Geometry check sheet. Reference: the model listing, model coordinates, mm. Coordinates: 2 decimals unless noted, no trailing zeros. Write each loop counter-clockwise with the first axis right and the second up, starting at its lowest first coordinate (ties: lowest second). Pieces come first, ordered by that corner, then holes. Notation, with made-up numbers: M 71,37 L 117,37 A15 ccw 117,61 Z; hole C -30,52 d7. An arc over 180 degrees is marked long. Put each result on its own line as item: value. Start each with the question number.
1) Cross-section at A-A on z = 0. Record the cut outline in (x, y) (3 decimals), plus the area to 3 significant figures.
2) Gauge pin test, flat ends, axial feed: pin 1 (8 mm diameter, centred on x = 1, y = -21, fed in from -Z); pin 2 (8 mm diameter, centred on x = -5.5, y = -5.5, fed in from -Z); pin 3 (12 mm diameter, centred on y = 16, z = 39, fed in from -X); pin 4 (3 mm diameter, centred on x = -15.5, z = -24.5, fed in from +Y). Record the tip position at first contact, or that the pin passes through.
3) Scan lines: line 1 along Z through (x, y) = (8, 0) (3 decimals); line 2 along Z through (x, y) = (15, -38.5); line 3 along Y through (x, z) = (12.5, 23.5). Record each from-to range of solid material in increasing order.
4) Mould release check, pull along Z, two halves, no side actions. Record for faces 1 (the flat face through (27, 22, -41)), 2 (the cylindrical face through (-0.36, -35.81, -27.46)), 3 (the conical face through (-26.854, -10.915, -49.155)): released by +Z, released by -Z, zero draft, split by the parting line, or undercut.
5) Cross-section at C-C on x = -11. Record the cut outline in (y, z) (3 decimals), plus the area to 3 significant figures.
from build123d import *

# Parameters (mm, degrees)
F0_R     = 52
F0_R_2   = 45.125
F1_DEPTH = 27
F2_SIZE  = 1
F3_SIZE2 = 1.7320508076
F3_SIZE  = 3


with BuildPart() as f1:
    # F0 (on Right) → F1 (new body, symmetric)
    with BuildSketch(Plane.YZ):
        Circle(F0_R)
        Circle(F0_R_2, mode=Mode.SUBTRACT)
    extrude(amount=F1_DEPTH, both=True)

    # F2
    f2_edges = [f1.edges().sort_by_distance(p)[0] for p in [
        (27, -45.125, 0),
        (-27, -45.125, 0),
    ]]
    chamfer(f2_edges, length=F2_SIZE)

    # F3
    f3_edges = [f1.edges().sort_by_distance(p)[0] for p in [
        (-27, -52, 0),
        (27, -52, 0),
    ]]
    f3_side = f1.faces().sort_by_distance((0, -52, 0))[0]
    chamfer(f3_edges, length=F3_SIZE, length2=F3_SIZE2, reference=f3_side)


solid = f1.part
Answer key:
1. outline: M -27,-50.268 L -24,-52 L 24,-52 L 27,-50.268 L 27,-46.125 L 26,-45.125 L -26,-45.125 L -27,-46.125 Z; M -27,46.125 L -26,45.125 L 26,45.125 L 27,46.125 L 27,50.268 L 24,52 L -24,52 L -27,50.268 Z
1. area: 730 mm²
2. pin 1: stops at z = -49.14
2. pin 2: stops at z = -51.98
2. pin 3: stops at x = -27
2. pin 4: stops at y = 46.64
3. line 1: z = -52 to -45.125, 45.125 to 52
3. line 2: z = -34.95 to -23.54, 23.54 to 34.95
3. line 3: y = -46.39 to -38.52, 38.52 to 46.39
4. face 1: zero draft
4. face 2: undercut
4. face 3: split by the parting line
5. outline: C 0,0 d104; hole C 0,0 d90.25
5. area: 2,100 mm²
